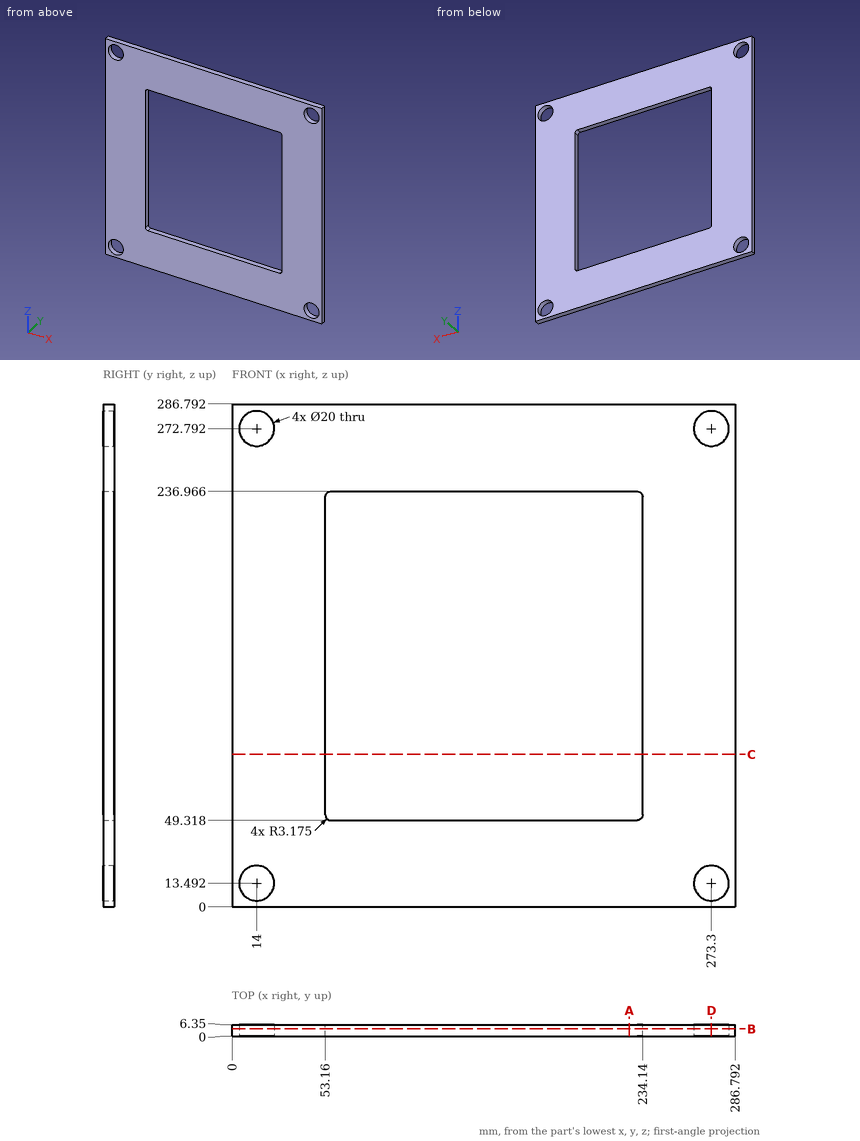
Study the drawing (mm; zero at the part's minimum x, y, z) and answer. Round coordinates to 2 decimals unless told otherwise and drop trailing zeros. Loops run counter-clockwise (first coordinate to the right, second up) from the corner with the lowest first, then second, coordinate; pieces in that order, holes last. Notation, with made-up numbers: (4, 63) -> (28, 63) arc R24 ccw to (28, 87) -> close; hole circle Ø1 at (19, 11.25). An arc over 180 degrees is marked (long way). Use one line per item in the form item = value.
1. The part is cut by section A-A on x = 226.5. Determine the outline of the cut face in (y, z).
Answer key:
outline = (0, 0) -> (6.35, 0) -> (6.35, 49.32) -> (0, 49.32) -> close; (0, 236.97) -> (6.35, 236.97) -> (6.35, 286.79) -> (0, 286.79) -> close
2. The part is cut by section D-D on x = 273.3. Determine the outline of the cut face in (y, z), and give its area (3 significant figures).
Answer key:
outline = (0, 0) -> (6.35, 0) -> (6.35, 3.49) -> (0, 3.49) -> close; (0, 23.49) -> (6.35, 23.49) -> (6.35, 262.79) -> (0, 262.79) -> close; (0, 282.79) -> (6.35, 282.79) -> (6.35, 286.79) -> (0, 286.79) -> close
area = 1,570 mm²
3. The part is cut by section C-C on z = 87. Determine the outline of the cut face in (x, y).
Answer key:
outline = (0, 0) -> (53.16, 0) -> (53.16, 6.35) -> (0, 6.35) -> close; (234.14, 0) -> (286.79, 0) -> (286.79, 6.35) -> (234.14, 6.35) -> close
4. The part is cut by section B-B on y = 4. Give the number of separate pieces and of enclosed holes in the cut face, and give its area (3 significant figures).
Answer key:
separate_pieces = 1
enclosed_holes = 5
area = 47,000 mm²
5. Find the intervals of material crossed by probe 1 along Z at (x, y) = (273.3, 4); probe 2 along X at (y, z) = (3.75, 166); probe 3 along Z at (x, y) = (63.5, 1), in increasing order. Write a range as [from, to].
Answer key:
probe_1 = [0, 3.49], [23.49, 262.79], [282.79, 286.79]
probe_2 = [0, 53.16], [234.14, 286.79]
probe_3 = [0, 49.32], [236.97, 286.79]
6. A flat-ended cylindrical pin translates along its axis: pin 1 Ø12 at (x, z) = (14, 13.492) entering from +Y. Find the tip coordinate at first contact, or state that the pin passes through.
Answer key:
pin_1 = through
